Drawing for the job (mm, zero at the part's lowest x, y, z). A direction names the side the tool comes from. Coordinates: 2 decimals unless noted, no trailing zeros. Loops run counter-clockwise (first coordinate to the right, second up) from the corner with the lowest first, then second, coordinate; pieces in that order, holes last.
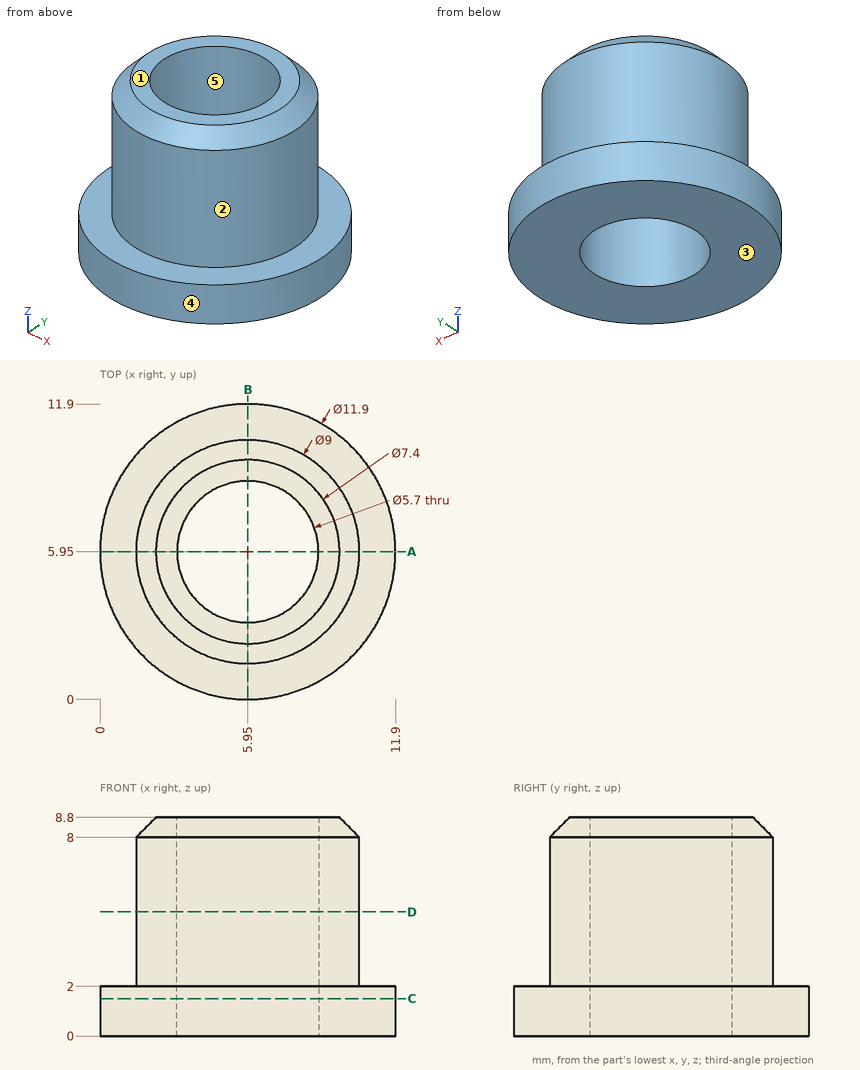
Q1. Mould opens along Y. For the marked faces 3, 4 and 5 say: released by +Y, released by -Y, zero draft, split by the parting line, or undercut.
Q2. Saw through at C-C (z = 1.5). List the corners of the cut face in (x, y).
Q3. Drop flat-ended pins along their axis: P1, Ø3, axis at y = 4.5, z = 7, coming from the +X side; P2, Ø1, axis at x = 5, z = 4, coming from the -Y side; P3, Ø5, axis at x = 5.95, y = 5.95, coming from the +Z side. Give the stop position or say it passes through.
Q4. Tool access for the marked faces 1 and 2: list every direction of +Z, -Z, +X, -X, +Y, -Y with a clear straight run to the whole face (end or side of a thin tool).
Q5. Saw through at A-A (y = 5.95). List the corners of the cut face in (x, z), plus the area to 3 significant figures.
Q6. Saw through at D-D (z = 5). List the corners of the cut face in (x, y), plus the area to 3 significant figures.
Q7. Probe line 1 (Y direction, x = 5.95, z = 3.25); line 2 (Z direction, x = 9.75, y = 9.25). List the from-to ranges inside material, lowest first.
Checked values:
1. face 3: zero draft
1. face 4: split by the parting line
1. face 5: undercut
2. outline: circle Ø11.9 at (5.95, 5.95); hole circle Ø5.7 at (5.95, 5.95)
3. P1: stops at x = 10.45
3. P2: stops at y = 1.47
3. P3: passes through
4. face 1: +Z, +X, -X, +Y, -Y
4. face 2: +Z
5. outline: (0, 0) - (3.1, 0) - (3.1, 8.8) - (2.25, 8.8) - (1.45, 8) - (1.45, 2) - (0, 2) - close; (8.8, 0) - (11.9, 0) - (11.9, 2) - (10.45, 2) - (10.45, 8) - (9.65, 8.8) - (8.8, 8.8) - close
5. area: 34.2 mm2
6. outline: circle Ø9 at (5.95, 5.95); hole circle Ø5.7 at (5.95, 5.95)
6. area: 38.1 mm2
7. line 1: y = 1.45 to 3.1, 8.8 to 10.45
7. line 2: z = 0 to 2
